Can you work these out from the model? Positions are in its coordinate system, mm. A direction names the side the tool comes from. Give positions to 0.01 mm unless a question says otherwise; leave off trailing zeros. Loops run counter-clockwise (first coordinate to the right, second up) from the corner with the lowest first, then second, coordinate; pieces in that order, holes last. Notation, with made-up numbers: (44, 50) -> (68, 50) arc R19 cw to (68, 63) -> close; hole circle Ø5 at (23, 69). An arc over 180 degrees is marked (long way). Return JSON: item names as keys, results as strings. Group by question number.
Q1. Suppose I cut it at C-C, the plane x = -40. Please give me the cut outline in (y, z).
Q2. Thinking about a two-plate mould opening in X: for faces 1 (the flat face through (-27.202, -24.248, 2.954)), 2 (the flat face through (-27.34, -25.05, 2.95)), 3 (the flat face through (-55, -40.777, 3)), which applies, pulls with the +X half, pulls with the -X half, needs draft (parallel to the pull), parting line crosses it, or undercut?
Q3. Will these pins go through, and if not, where does the flat tip stop? pin 1 (6 mm diameter, centred on x = -52.5, z = -16.5, fed in from +Y); pin 2 (3 mm diameter, centred on y = -17, z = -28, fed in from +X); pin 3 (10 mm diameter, centred on x = -34, y = -36, fed in from -Z); pin 4 (10 mm diameter, centred on y = -10, z = 135, fed in from +X).
Q4. Suppose I cut it at B-B, the plane z = 72.5. Please give me the cut outline in (x, y), and give its area (3 significant figures).
Q5. Suppose I cut it at A-A, the plane y = -32. Please give me the cut outline in (x, z), and give its area (3 significant figures).
Q6. Which directions (+Z, -Z, +X, -X, +Y, -Y) give clear straight access to the entire face, cutting with the end or side of a thin tool? Please do faces 4 (the flat face through (26.864, -24.617, 2.954)), 5 (the flat face through (58, -40.277, 3)), 6 (the flat face through (-55, -40.277, 3)).
Q7. I need wall thicknesses on line 1 along Z through (x, y) = (55.5, -40.6); line 2 along Y through (x, z) = (68, -192.5); line 3 along X through (y, z) = (-40.6, 201). Which ranges of each line are inside material? Lowest first, please. Write a range as [from, to].
```python
from build123d import *

# Parameters (mm, degrees)
BASE_FLANGE1_DEPTH = 211
SKETCH13_R         = 6.1
EXTRUDE1_DEPTH     = 0.5
SKETCH16_R         = 1.75
EXTRUDE2_DEPTH     = 0.5
SKETCH17_R         = 1.75
EXTRUDE3_DEPTH     = 0.5
SKETCH18_R         = 1.75
EXTRUDE4_DEPTH     = 0.5
HEM1_START         = -211
HEM1_DEPTH         = 422
HEM1_2_DEPTH       = 422


# Read off the part's stored shape, not the designer's step: Hem1
# Sheet-metal steps are written as plain solids
with BuildPart() as part:
    # Sketch1 → Base-Flange1 (new, symmetric)
    with BuildSketch(Plane.XY):
        with BuildLine():
            Line((-64.5, -40.776737244), (-45.083318098, -40.776737244))
            ThreePointArc((-45.083318098, -40.776737244), (-44.53966104, -40.674749048), (-44.069932786, -40.382653249))
            Line((-44.069932786, -40.382653249), (-10.133853114, -9.285965521))
            ThreePointArc((-10.133853114, -9.285965521), (0, -5.345125574), (10.133853114, -9.285965521))
            Line((10.133853114, -9.285965521), (44.069932786, -40.382653249))
            ThreePointArc((44.069932786, -40.382653249), (44.53966104, -40.674749048), (45.083318098, -40.776737244))
            Line((45.083318098, -40.776737244), (73.5, -40.776737244))
            Line((73.5, -40.776737244), (73.5, -40.276737244))
            Line((73.5, -40.276737244), (45.083318098, -40.276737244))
            ThreePointArc((45.083318098, -40.276737244), (44.720880059, -40.208745113), (44.40772789, -40.014014581))
            Line((44.40772789, -40.014014581), (10.471648218, -8.917326853))
            ThreePointArc((10.471648218, -8.917326853), (0, -4.845125574), (-10.471648218, -8.917326853))
            Line((-10.471648218, -8.917326853), (-44.40772789, -40.014014581))
            ThreePointArc((-44.40772789, -40.014014581), (-44.720880059, -40.208745113), (-45.083318098, -40.276737244))
            Line((-45.083318098, -40.276737244), (-64.5, -40.276737244))
            Line((-64.5, -40.276737244), (-64.5, -40.776737244))
        make_face()
    extrude(amount=BASE_FLANGE1_DEPTH, both=True)

    # Sketch13 → Extrude1 (cut)
    with BuildSketch(Plane(origin=(0, -40.276737244, 0), x_dir=(1, 0, 0), z_dir=(0, 1, 0))):
        with Locations(Location((-54.791659049, 201, 0), (0, 0, 180))):
            Circle(SKETCH13_R)
        with Locations(Location((55.5, 201, 0), (0, 0, 180))):
            Circle(SKETCH13_R)
        with Locations((55.5, -201)):
            Circle(SKETCH13_R)
        with Locations((-54.791659049, -201)):
            Circle(SKETCH13_R)
    extrude(amount=-EXTRUDE1_DEPTH, mode=Mode.SUBTRACT)

    # Sketch16 → Extrude2 (cut)
    with BuildSketch(Plane(origin=(0.337795104, 0.368638668, 0), x_dir=(0, 0, -1), z_dir=(0.6755902076156584, 0.7372773368101257, 0))):
        with Locations(Location((-196, -16.74496761, 0), (0, 0, 90))):
            Circle(SKETCH16_R)
        with Locations(Location((196, -16.74496761, 0), (0, 0, 270))):
            Circle(SKETCH16_R)
        with Locations(Location((0, -16.74496761, 0), (0, 0, 90))):
            Circle(SKETCH16_R)
    extrude(amount=-EXTRUDE2_DEPTH, mode=Mode.SUBTRACT)

    # Sketch17 → Extrude3 (cut)
    with BuildSketch(Plane(origin=(0, -40.276737244, 0), x_dir=(1, 0, 0), z_dir=(0, 1, 0))):
        with Locations(Location((55.5, 0, 0), (0, 0, 180))):
            Circle(SKETCH17_R)
    extrude(amount=-EXTRUDE3_DEPTH, mode=Mode.SUBTRACT)

    # Sketch18 → Extrude4 (cut)
    with BuildSketch(Plane(origin=(0, -40.276737244, 0), x_dir=(1, 0, 0), z_dir=(0, 1, 0))):
        with Locations(Location((55.5, -184, 0), (0, 0, 180))):
            Circle(SKETCH18_R)
        with Locations((55.5, 184)):
            Circle(SKETCH18_R)
    extrude(amount=-EXTRUDE4_DEPTH, mode=Mode.SUBTRACT)

    # Hem1 outline → Hem1 (cut)
    with BuildSketch(Plane.XY.offset(HEM1_START)):
        with BuildLine():
            Line((73.5, -40.276737244), (72.664213562, -40.276737244))
            ThreePointArc((72.664213562, -40.276737244), (72, -40.648057588), (71.25, -40.776737244))
            Line((71.25, -40.776737244), (73.5, -40.776737244))
            Line((73.5, -40.776737244), (73.5, -40.276737244))
        make_face()
    extrude(amount=HEM1_DEPTH, mode=Mode.SUBTRACT)

    # Hem1 2 outline → Hem1 2 (add)
    with BuildSketch(Plane.XY.offset(HEM1_START)):
        with BuildLine():
            Line((66.5, -36.276737244), (66.5, -36.776737244))
            Line((66.5, -36.776737244), (71.25, -36.776737244))
            ThreePointArc((71.25, -36.776737244), (73, -38.526737244), (71.25, -40.276737244))
            Line((71.25, -40.276737244), (72.664213562, -40.276737244))
            ThreePointArc((72.664213562, -40.276737244), (73.371320344, -37.776737244), (71.25, -36.276737244))
            Line((71.25, -36.276737244), (66.5, -36.276737244))
        make_face()
    extrude(amount=HEM1_2_DEPTH)


solid = part.part
```
Ans:
{
 "1": {"outline": "(-36.65, -211) -> (-35.98, -211) -> (-35.98, 211) -> (-36.65, 211) -> close"},
 "2": {"face 1": "pulls with the -X half", "face 2": "undercut", "face 3": "needs draft"},
 "3": {"pin 1": "stops at y = -40.28", "pin 2": "stops at x = 20.93", "pin 3": "stops at z = -211", "pin 4": "stops at x = 17.11"},
 "4": {"outline": "(-64.5, -40.78) -> (-45.08, -40.78) arc R1.5 ccw to (-44.07, -40.38) -> (-10.13, -9.29) arc R15 cw to (10.13, -9.29) -> (44.07, -40.38) arc R1.5 ccw to (45.08, -40.78) -> (71.25, -40.78) arc R2.25 ccw to (71.25, -36.28) -> (66.5, -36.28) -> (66.5, -36.78) -> (71.25, -36.78) arc R1.75 cw to (71.25, -40.28) -> (45.08, -40.28) arc R1 cw to (44.41, -40.01) -> (10.47, -8.92) arc R15.5 ccw to (-10.47, -8.92) -> (-44.41, -40.01) arc R1 cw to (-45.08, -40.28) -> (-64.5, -40.28) -> close", "area": "86.6 mm^2"},
 "5": {"outline": "(-35.66, -211) -> (-34.92, -211) -> (-34.92, 211) -> (-35.66, 211) -> close; (34.92, -211) -> (35.66, -211) -> (35.66, 211) -> (34.92, 211) -> close", "area": "625 mm^2"},
 "6": {"face 4": "+Z, -Z, -Y", "face 5": "+Z, -Z", "face 6": "+Z, -Z, -X, +Y"},
 "7": {"line 1": "z = [-211, -207.1], [-194.9, -185.75], [-182.25, -1.75], [1.75, 182.25], [185.75, 194.9], [207.1, 211]", "line 2": "y = [-40.78, -40.28], [-36.78, -36.28]", "line 3": "x = [-64.5, -60.89], [-48.69, -44.38], [44.38, 49.4], [61.6, 72.12]"}
}
